For this review, use the dimensioned drawing (mm, ordinates from the lowest corner) and the shaded views. A direction names the side the tool comes from. Give positions to 0.01 mm unless a question says otherwise; leave off trailing zeros. Order: outer loops, then holes, each group sorted by start corner. A loop starts at its lowest first (then second) coordinate and runs counter-clockwise, first axis right, second up. Notation, with made-up numbers: (-20, 58.5) -> (5, 58.5) arc R18 ccw to (5, 64.5) -> close; hole circle Ø11 at (75.5, 59). An arc over 180 degrees is marked (long way). Answer as a JSON object with one key per item and string values. Group by question number.
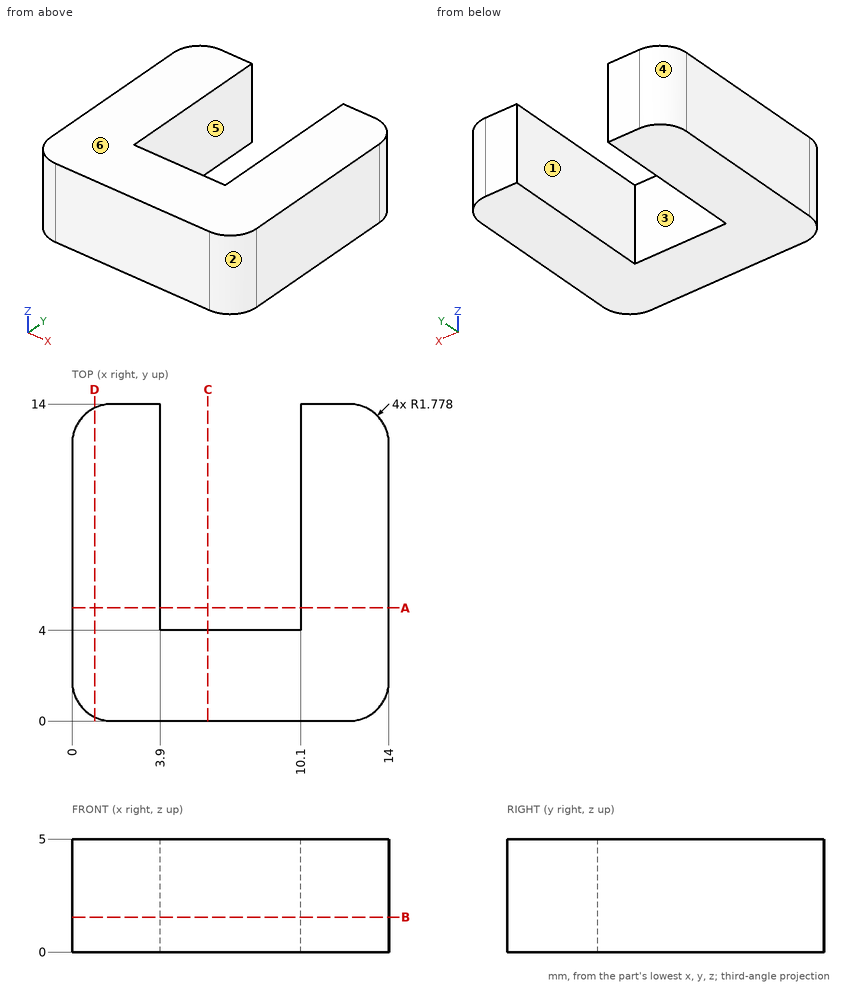
1. Draft analysis for pull direction X (two halves, no side actions). For the marked faces 1, 2, 3 and 4, state which applies: pulls with the +X half, pulls with the -X half, needs draft (parallel to the pull), parting line crosses it, or undercut.
2. For pin 1 (1.5 mm diameter, centred on x = 6, z = 3.5, fed in from +Y), flat-tipped, find the tip position at first contact; note if it passes through.
3. Machinability: for the marked faces 5 and 6, which of the approach directions +Z, -Z, +X, -X, +Y, -Y give a long, thin tool a straight path to every point of the face, cutting with its end or side? Answer none if there is none.
4. Take a section at C-C on x = 6. Give the boundary of the cut face in (y, z).
5. Take a section at D-D on x = 1. Give the boundary of the cut face in (y, z).
6. Take a section at B-B on z = 1.55. Give the boundary of the cut face in (x, y).
7. For probe 1 along X at (y, z) = (12, 2.3); probe 2 along Y at (x, z) = (5.5, 4.25); probe 3 along X at (y, z) = (13, 0.6), list the stretches that pass through material, from the lowest coordinate up. Write a range as [from, to].
8. Take a section at A-A on y = 5. Give the boundary of the cut face in (x, z).
Checks:
{
 "1": {"face 1": "undercut", "face 2": "pulls with the +X half", "face 3": "undercut", "face 4": "pulls with the -X half"},
 "2": {"pin 1": "stops at y = 4"},
 "3": {"face 5": "+Z, -Z, +Y", "face 6": "+Z, +X, -X, +Y, -Y"},
 "4": {"outline": "(0, 0) -> (4, 0) -> (4, 5) -> (0, 5) -> close"},
 "5": {"outline": "(0.18, 0) -> (13.82, 0) -> (13.82, 5) -> (0.18, 5) -> close"},
 "6": {"outline": "(0, 1.78) arc R1.78 ccw to (1.78, 0) -> (12.22, 0) arc R1.78 ccw to (14, 1.78) -> (14, 12.22) arc R1.78 ccw to (12.22, 14) -> (10.1, 14) -> (10.1, 4) -> (3.9, 4) -> (3.9, 14) -> (1.78, 14) arc R1.78 ccw to (0, 12.22) -> close"},
 "7": {"probe 1": "x = [0, 3.9], [10.1, 14]", "probe 2": "y = [0, 4]", "probe 3": "x = [0.18, 3.9], [10.1, 13.82]"},
 "8": {"outline": "(0, 0) -> (3.9, 0) -> (3.9, 5) -> (0, 5) -> close; (10.1, 0) -> (14, 0) -> (14, 5) -> (10.1, 5) -> close"}
}
